Model file for the job. Use its own axes, mm. Face numbers are marked on the shaded views. A direction names the side the tool comes from. Round coordinates to 2 decimals unless told otherwise and drop trailing zeros. Loops run counter-clockwise (first coordinate to the right, second up) from the corner with the lowest first, then second, coordinate; pieces in that order, holes last. Notation, with made-up numbers: M -17,-13.5 L 34,-13.5 A25 ccw 34,8.5 Z; hole C 58,-35.5 d3. An arc over 180 degrees is marked long. Answer in a Markdown table with one row per item.
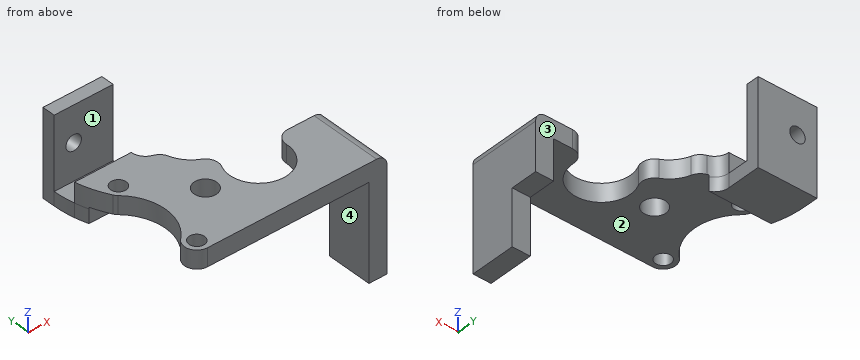
Autodesk Inventor part; units mm, degrees
ref_plane "YZ Plane" through (0, 0, 0) normal (1, 0, 0) x (0, 1, 0)
ref_plane "XZ Plane" through (0, 0, 0) normal (0, 1, 0) x (-1, 0, 0)
ref_plane "XY Plane" through (0, 0, 0) normal (0, 0, 1) x (1, 0, 0)
sketch "Sketch1" plane through (0, 0, 0) normal (0, 0, 1) x (1, 0, 0)
  circle A0 centre (-13, 8.75) radius 1.5
  circle A1 centre (-3.75, 0) radius 2 construction
  circle A2 centre (-13, -8.75) radius 1.5
  arc A3 (4.5834, 1.85) -> (4.5834, -1.85) centre (6.55, 0) ccw construction
  arc A4 (4.8736, 5.3432) -> (1.4897, 2.3987) centre (6.55, 0) ccw construction
  circle A5 centre (-3.75, 0) radius 2.2
  arc A6 (-14.5962, -6.9913) -> (-14.5962, 6.9913) centre (-20.9415, 0) ccw
  arc A7 (-13, 11.125) -> (-15.0744, 7.5935) centre (-13, 8.75) ccw construction
  line L0 (14.125, 11.125) -> (-18.25, 11.125)
  line L1 (-18.25, -11.125) -> (14.125, -11.125)
  arc A8 (-14.5962, -6.9913) -> (-13, -11.125) centre (-13, -8.75) ccw
  line L2 (-11.5, 8.75) -> (-11.5, -8.75) construction
  line L3 (21.75, 2.8432) -> (21.75, -11.125)
  line L4 (21.75, -11.125) -> (14.125, -11.125)
  line L5 (14.125, -11.125) -> (14.125, 11.125) construction
  line L6 (18.25, -7) -> (18.25, 7) construction
  arc A9 (-3, 11.125) -> (-2.7358, 9.3552) centre (3.0597, 11.125) ccw construction
  arc A10 (-2.7358, 9.3552) -> (-4.3762, 11.0097) centre (-5.1268, 8.625) ccw
  arc A11 (-2.7358, 9.3552) -> (0.349, 5.7054) centre (3.0597, 11.125) ccw
  line L7 (11.3745, 2.8432) -> (14.6427, 2.8432) construction
  arc A12 (11.3745, 2.8432) -> (4.8736, 5.3432) centre (6.55, 0) ccw construction
  arc A13 (1.4897, 2.3987) -> (0.349, 5.7054) centre (-0.7693, 3.4695) ccw
  arc A14 (0.349, 5.7054) -> (4.8736, 5.3432) centre (3.0597, 11.125) ccw construction
  arc A15 (1.4897, 2.3987) -> (12.145, 0.2373) centre (6.55, 0) ccw
  arc A16 (14.6427, 2.8432) -> (12.145, 0.2373) centre (14.6427, 0.3432) ccw
  arc A17 (12.145, 0.2373) -> (11.3745, 2.8432) centre (6.55, 0) ccw construction
  line L8 (14.6427, 2.8432) -> (21.75, 2.8432)
  line L9 (-12.425, 16.375) -> (-15.425, 16.375)
  line L10 (-15.425, 17.675) -> (-12.425, 17.675)
  line L11 (-15.425, 17.675) -> (-17.6949, 17.675)
  line L12 (-12.425, 17.675) -> (-6.2949, 17.675)
  line L13 (-6.2949, 17.675) -> (-6.2949, 20.175)
  line L14 (-6.2949, 20.175) -> (-17.6949, 20.175)
  line L15 (-17.6949, 20.175) -> (-17.6949, 17.675)
  arc A18 (-17.6949, 17.675) -> (-15.0744, 7.5935) centre (3.0083, 17.675) ccw
  line L16 (-6.2949, 13.625) -> (-17.2949, 13.625)
  line L17 (-6.2949, 13.625) -> (-6.2949, 17.675)
  arc A19 (-6.2949, 13.625) -> (-4.3762, 11.0097) centre (-3.553, 13.625) ccw
  arc A20 (-4.3762, 11.0097) -> (-5.1268, 11.125) centre (-5.1268, 8.625) ccw construction
  arc A21 (-15.0744, 7.5935) -> (-14.5962, 6.9913) centre (-13, 8.75) ccw
  point P0 (0, 0)
  point P1 (-4.6789, 11.125)
  point P2 (-16.6314, 11.125)
  dimension "d0" = 0.2
  dimension "d1" = 2.5
  dimension "d3" = 3.5
  dimension "d4" = 10
  dimension "d5" = 2.5
  dimension "d6" = 2.5
  dimension "d7" = 2.5
  dimension "d8" = 2.5
  dimension "d16" = 2.5
  dimension "d17" = 2.5
  dimension "d18" = 11
  dimension "d19" = 11.4
extrude "Extrusion1" add sketch "Sketch1" along normal blind 3.5 contours A6 A21 A18 L0 A19 A10 A11 A13 A15 A16 L8 L3 L4 L1 A8 | A18 L16 A19 L0
sketch "Sketch2" plane through (0, 0, 0) normal (0, 0, -1) x (-1, 0, 0)
  line L0 (-18.25, 7) -> (-18.25, -7)
  line L1 (-21.75, -11.125) -> (-21.75, 2.8432)
  line L2 (-18.25, -7) -> (-18.25, -11.125)
  line L3 (13, -11.125) -> (-21.75, -11.125)
  line L4 (-18.25, -11.125) -> (-21.75, -11.125)
  line L5 (-21.75, 2.8432) -> (-14.6427, 2.8432)
  line L6 (-21.75, 2.8432) -> (-18.25, 2.8432)
  point P0 (0, 0)
extrude "Extrusion2" add sketch "Sketch2" along normal blind 18.55
fillet "Fillet1" radius 2 1 edges at (21.75, -4.1409, 3.5)
extrude "Extrusion3" add sketch "Sketch1" against normal blind 0.325 contours A18 L16 A19 L0
sketch "Sketch5" plane through (0, 0, -0.325) normal (0, 0, -1) x (-1, 0, 0)
  line L0 (17.2949, 13.625) -> (6.2949, 13.625)
  arc A0 (4.6789, 11.125) -> (6.2949, 13.625) centre (3.553, 13.625) ccw
  line L1 (4.6789, 11.125) -> (16.6314, 11.125)
  arc A1 (16.6314, 11.125) -> (17.2949, 13.625) centre (-3.0083, 17.675) ccw
  line L2 (6.2949, 13.625) -> (6.2949, 17.675)
  line L3 (6.2949, 17.675) -> (6.2949, 20.175)
  line L4 (6.2949, 20.175) -> (17.6949, 20.175)
  line L5 (17.6949, 20.175) -> (17.6949, 17.675)
  line L6 (12.425, 17.675) -> (6.2949, 17.675)
  line L7 (15.425, 17.675) -> (12.425, 17.675)
  line L8 (15.425, 17.675) -> (17.6949, 17.675)
  arc A2 (15.0744, 7.5935) -> (17.6949, 17.675) centre (-3.0083, 17.675) ccw
  line L9 (6.2949, 13.625) -> (17.2949, 13.625)
  point P0 (0, 0)
extrude "Extrusion4" add sketch "Sketch5" along normal blind 2.675
extrude "Extrusion5" add sketch "Sketch5" against normal blind 14 contours L8 L7 L6 L3 L4 L5
sketch "Sketch6" plane through (-17.6949, 17.675, -0.325) normal (0, -1, 0) x (1, 0, 0)
  circle A0 centre (3.7699, 7.075) radius 1.5
  point P0 (17.6949, 0.325)
extrude "Extrusion6" cut sketch "Sketch6" against normal blind 14
sketch "Sketch7" plane through (21.75, -11.125, -18.55) normal (1, 0, 0) x (0, 0, -1)
  line L0 (-10.8, 13.75) -> (-10.8, 8.75)
  line L1 (-10.8, 13.75) -> (-10.8, 13.9682)
  line L2 (-18.55, 13.9682) -> (0, 13.9682)
  line L3 (-10.8, 8.75) -> (0, 8.75)
  line L4 (0, 0) -> (0, 13.9682)
  line L5 (0, 8.75) -> (0, 13.9682)
  point P0 (-18.55, 11.125)
extrude "Extrusion7" cut sketch "Sketch7" against normal blind 10
properties part number "MotorEncoderBracket"
1. Saw through at C-C (x = -9.5). Write the cut outline in (y, z) (3 decimals).
Verdict:
| item | result |
|---|---|
| outline | M -11.125,0 L 11.125,0 L 11.125,-3 L 20.175,-3 L 20.175,13.675 L 17.675,13.675 L 17.675,-0.325 L 13.625,-0.325 L 13.625,3.5 L -11.125,3.5 Z |
2. Saw through at D-D (y = -4). Write the cut outline in (x, z), and give its area (3 significant figures).
Verdict:
| item | result |
|---|---|
| outline | M -12.39,0 L 2.63,0 L 2.63,3.5 L -12.39,3.5 Z; M 10.47,0 L 18.25,0 L 18.25,-18.55 L 21.75,-18.55 L 21.75,1.5 A2 ccw 19.75,3.5 L 10.47,3.5 Z |
| area | 156 mm² |
3. Saw through at A-A (z = 2). State how many separate pieces and enclosed holes the cut face has, and give its area (3 significant figures).
Verdict:
| item | result |
|---|---|
| separate pieces | 2 |
| enclosed holes | 3 |
| area | 542 mm² |
4. Pin check, flat tips, straight feed: pin 1 (8 mm diameter, centred on x = -11, z = 4.5, fed in from -Y) (3 decimals); pin 2 (13 mm diameter, centred on x = 6.55, y = 0, fed in from -Z); pin 3 (3 mm diameter, centred on x = -10, y = 15, fed in from +Z); pin 4 (18 mm diameter, centred on x = -6.5, y = 3.5, fed in from -Z). Stop position of each tip, or through.
Verdict:
| item | result |
|---|---|
| pin 1 | stops at y = -11.125 |
| pin 2 | stops at z = 0 |
| pin 3 | stops at z = 3.5 |
| pin 4 | stops at z = -3 |
5. Saw through at B-B (z = 6.75). Write the cut outline in (x, y) (3 decimals), and give its area (3 significant figures).
Verdict:
| item | result |
|---|---|
| outline | M -17.695,17.675 L -15.425,17.675 L -15.425,20.175 L -17.695,20.175 Z; M -12.425,17.675 L -6.295,17.675 L -6.295,20.175 L -12.425,20.175 Z |
| area | 21.0 mm² |
6. Tool access for the marked faces 1, 2, 3 and 4: list every direction of +Z, -Z, +X, -X, +Y, -Y with a clear straight run to the whole face (end or side of a thin tool).
Verdict:
| item | result |
|---|---|
| face 1 | +Z, +X, -X |
| face 2 | -Z, -X, -Y |
| face 3 | +Z, -Z, +X, +Y |
| face 4 | -Z, -X, +Y, -Y |
7. Wall check: probe 1 along Y at (x, z) = (-13, 1) (3 decimals); probe 2 along Z at (x, y) = (17.5, -1); probe 3 along X at (y, z) = (-1.5, -5). Give the ranges that are in metal, low to high.
Verdict:
| item | result |
|---|---|
| probe 1 | y = -11.125 to -10.25, -7.25 to -5.106, 5.106 to 7.25, 10.25 to 13.625, 17.675 to 20.175 |
| probe 2 | z = 0 to 3.5 |
| probe 3 | x = 18.25 to 21.75 |
